Print and shaded views of the part. All mm, measured from the part's lowest x, y and z. A direction names the side the tool comes from. Give positions to 0.01 mm unless a question says otherwise; leave off trailing zeros. Loops run counter-clockwise (first coordinate to the right, second up) from the corner with the lowest first, then second, coordinate; pieces in that order, holes last. Notation, with made-up numbers: (-8.5, 10) - (15.5, 10) arc R24 cw to (15.5, 21) - close; hole circle Ø7 at (58.25, 78.5). An arc over 180 degrees is marked (long way). Return JSON: item names as keys, results as strings.
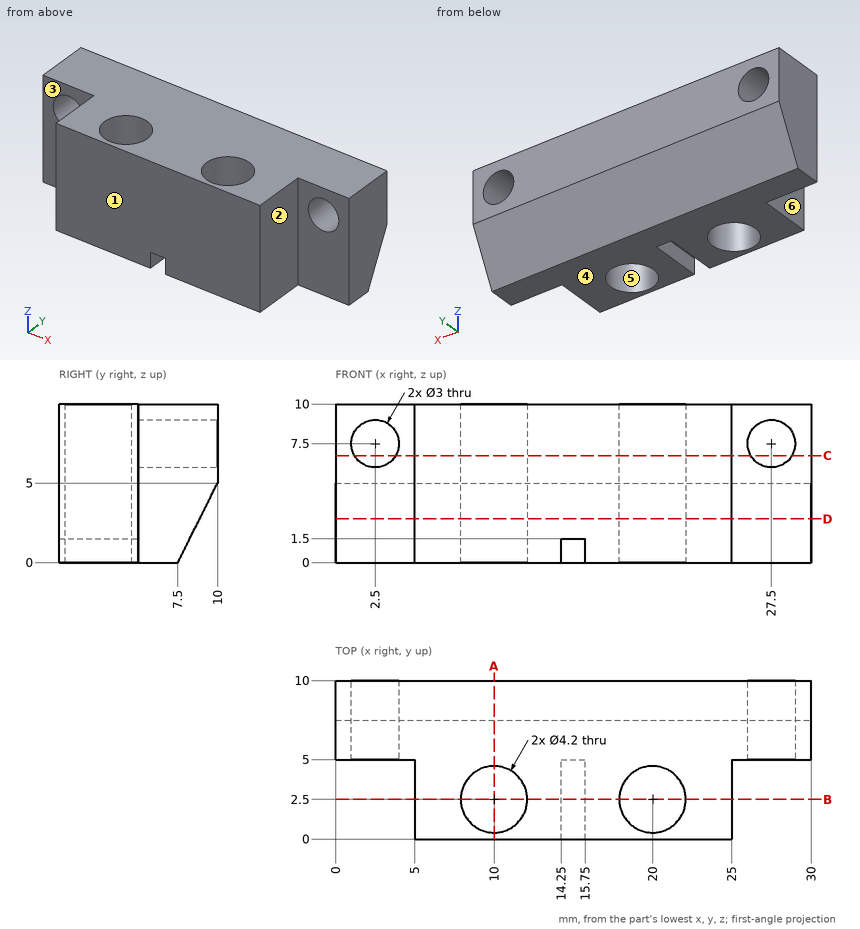
1. Cut at B-B, the plane y = 2.5. Write the cut outline in (x, z), plus the area to 3 significant figures.
Values follow:
{"outline": "(5, 0) - (7.9, 0) - (7.9, 10) - (5, 10) - close; (12.1, 0) - (14.25, 0) - (14.25, 1.5) - (15.75, 1.5) - (15.75, 0) - (17.9, 0) - (17.9, 10) - (12.1, 10) - close; (22.1, 0) - (25, 0) - (25, 10) - (22.1, 10) - close", "area": "114 mm²"}
2. Drop flat-ended pins along their axis: P1, Ø5, axis at x = 4.5, y = 2, coming from the +Z side; P2, Ø4, axis at y = 2, z = 6, coming from the +X side; P3, Ø1.5, axis at x = 3.5, z = 2.5, coming from the -Y side; P4, Ø0.8, axis at y = 3, z = 0.5, coming from the -X side. Give the stop position or say it passes through.
Values follow:
{"P1": "stops at z = 10", "P2": "stops at x = 25", "P3": "stops at y = 5", "P4": "stops at x = 5"}
3. Which spindle directions (+Z, -Z, +X, -X, +Y, -Y) get a long thin tool onto all of the face, cutting with end or side? Do the marked faces 1, 2 and 3. Say none if no direction does.
Values follow:
{"face 1": "+Z, -Z, +X, -X, -Y", "face 2": "+Z, -Z, +X, -Y", "face 3": "+Z, -Z, -X, -Y"}
4. Cut at D-D, the plane z = 2.75. Write the cut outline in (x, y) (3 decimals), plus the area to 3 significant figures.
Values follow:
{"outline": "(0, 5) - (5, 5) - (5, 0) - (25, 0) - (25, 5) - (30, 5) - (30, 8.875) - (0, 8.875) - close; hole circle Ø4.2 at (10, 2.5); hole circle Ø4.2 at (20, 2.5)", "area": "189 mm²"}
5. Drill centre lines: probe 1 along X at (y, z) = (6.35, 7.5); probe 2 along X at (y, z) = (4.25, 8.5); probe 3 along Z at (x, y) = (27.5, 7.1). Where is each one in solid material? Low to high.
Values follow:
{"probe 1": "x = 0 to 1, 4 to 26, 29 to 30", "probe 2": "x = 5 to 8.84, 11.16 to 18.84, 21.16 to 25", "probe 3": "z = 0 to 6, 9 to 10"}
6. Pull direction X, two halves, no side cores. Call the marked faces 4, 5 and 6: +X half, -X half, draft (parallel to the pull), parting line (faces both ways), or undercut.
Values follow:
{"face 4": "draft", "face 5": "undercut", "face 6": "-X half"}
7. Cut at C-C, the plane z = 6.75. Write the cut outline in (x, y), plus the area to 3 significant figures.
Values follow:
{"outline": "(0, 5) - (1.2, 5) - (1.2, 10) - (0, 10) - close; (3.8, 5) - (5, 5) - (5, 0) - (25, 0) - (25, 5) - (26.2, 5) - (26.2, 10) - (3.8, 10) - close; (28.8, 5) - (30, 5) - (30, 10) - (28.8, 10) - close; hole circle Ø4.2 at (10, 2.5); hole circle Ø4.2 at (20, 2.5)", "area": "196 mm²"}
8. Cut at A-A, the plane x = 10. Write the cut outline in (y, z), plus the area to 4 significant figures.
Values follow:
{"outline": "(0, 0) - (0.4, 0) - (0.4, 10) - (0, 10) - close; (4.6, 0) - (7.5, 0) - (10, 5) - (10, 10) - (4.6, 10) - close", "area": "51.75 mm²"}
